Check sheet for the modelled part. Datum: model origin and axes. Units: mm. A direction names the side the tool comes from. Give positions to 0.01 mm unless a question says otherwise; leave off trailing zeros. Loops run counter-clockwise (first coordinate to the right, second up) from the corner with the lowest first, then second, coordinate; pieces in that order, holes last. Notation, with made-up numbers: (-7, 23.5) - (52, 23.5) arc R9 ccw to (52, 29.5) - close; hole circle Ø8 at (83, -22). An arc over 180 degrees is marked (long way). Answer in a Markdown table with one row per item. Add a question column.
(1) Draft check along Z on faces 1 (the face through (0, 0, -1.778)), 2 (the face through (1.433, 8.476, -2.711)), 3 (the face through (0.95, 0.3, 36.53)), 4 (the face through (-1.433, -8.476, -2.711)). Enter one of: released by +Z, released by -Z, zero draft, split by the parting line, or undercut.
(2) Go/stop test with flat-tipped pins: P1, Ø4, axis at y = -8.5, z = 24.5, coming from the +X side; P2, Ø1.7, axis at y = 9.11, z = -2.79, coming from the +X side; P3, Ø3, axis at x = -9, z = 13.5, coming from the -Y side; P4, Ø5, axis at y = 6.5, z = 34.5, coming from the +X side. Record where each tip stops, or that it passes through.
(3) Set-up check for faces 5 (the face through (1, 1, 32.715)), 6 (the face through (-1.27, -9, -1)), 7 (the face through (0, 0, 40.97)): record each of +Z, -Z, +X, -X, +Y, -Y from which the full face is reachable in a straight line by a thin tool's end or side.
(4) Sectioned sample at A-A on z = 14.5. Enter the section's corners in (x, y), then the cut area to 3 significant figures.
(5) Thickness scan on L1, parallel to Y at x = 0, z = 0.35; L2, parallel to Z at x = 3.75, y = 10; L3, parallel to X at y = -0.5, z = 6. Record the ranges inside material, lowest first.
from build123d import *

# Parameters (mm, degrees)
SKETCH1_R           = 12.192
BOSS_EXTRUDE1_DEPTH = 30.8102
SKETCH2_R           = 0.99695
BOSS_EXTRUDE3_DEPTH = 10.16
SKETCH6_R           = 3.2004
BOSS_EXTRUDE4_DEPTH = 1.905
FILLET2_R           = 0.508
FILLET3_R           = 1.27
SKETCH7_R           = 11.7094
CUT_EXTRUDE1_DEPTH  = 1.016
SKETCH10_R          = 3.2258
BOSS_EXTRUDE5_DEPTH = 2.794
FILLET4_R           = 0.889
SKETCH11_W          = 0.3302
SKETCH11_H          = 2.1082
BOSS_EXTRUDE6_DEPTH = 5.08
SKETCH12_R          = 0.635
CUT_EXTRUDE2_DEPTH  = 0.3302
CIRPATTERN1_COUNT   = 2


with BuildPart() as part:
    # Sketch1 → Boss-Extrude1 (new body)
    with BuildSketch(Plane.XY):
        Circle(SKETCH1_R)
    extrude(amount=BOSS_EXTRUDE1_DEPTH)

    # Sketch2 → Boss-Extrude3 (add)
    with BuildSketch(Plane.XY.offset(30.8102)):
        Circle(SKETCH2_R)
    extrude(amount=BOSS_EXTRUDE3_DEPTH)

    # Sketch6 → Boss-Extrude4 (add)
    with BuildSketch(Plane.XY.offset(30.8102)):
        Circle(SKETCH6_R)
    extrude(amount=BOSS_EXTRUDE4_DEPTH)

    # Fillet2
    fillet2_edges = [part.edges().sort_by_distance(p)[0] for p in [
        (-0.99695, 0, 40.9702),
    ]]
    fillet(fillet2_edges, radius=FILLET2_R)

    # Fillet3
    fillet3_edges = [part.edges().sort_by_distance(p)[0] for p in [
        (-12.192, 0, 30.8102),
    ]]
    fillet(fillet3_edges, radius=FILLET3_R)

    # Sketch7 → Cut-Extrude1 (cut)
    with BuildSketch(Plane(origin=(0, 0, 0), x_dir=(-1, 0, 0), z_dir=(0, 0, -1))):
        Circle(SKETCH7_R)
    extrude(amount=-CUT_EXTRUDE1_DEPTH, mode=Mode.SUBTRACT)

    # Sketch10 → Boss-Extrude5 (add)
    with BuildSketch(Plane(origin=(0, 0, 1.016), x_dir=(-1, 0, 0), z_dir=(0, 0, -1))):
        Circle(SKETCH10_R)
    extrude(amount=BOSS_EXTRUDE5_DEPTH)

    # Fillet4
    fillet4_edges = [part.edges().sort_by_distance(p)[0] for p in [
        (3.2258, 0, -1.778),
    ]]
    fillet(fillet4_edges, radius=FILLET4_R)

    # Sketch11 → Boss-Extrude6 (add)
    with BuildSketch(Plane(origin=(0, 0, 1.016), x_dir=(-1, 0, 0), z_dir=(0, 0, -1))):
        with Locations((1.4351, -9.1059)):
            Rectangle(SKETCH11_W, SKETCH11_H)
    boss_extrude6 = extrude(amount=BOSS_EXTRUDE6_DEPTH)

    # Sketch12 → Cut-Extrude2 (cut)
    with BuildSketch(Plane(origin=(-1.27, 0, 0), x_dir=(0, 0, -1), z_dir=(1, 0, 0))):
        with Locations((2.794, -9.1059)):
            Circle(SKETCH12_R)
        Polygon((3.302, -8.0518), (4.064, -8.8138), (4.064, -8.0518), align=None)
        Polygon((4.064, -9.398), (3.302, -10.16), (4.064, -10.16), align=None)
    cut_extrude2 = extrude(amount=-CUT_EXTRUDE2_DEPTH, mode=Mode.SUBTRACT)

    # CirPattern1: Boss-Extrude6, Cut-Extrude2 ×2 about axis
    cirpattern1_axis = Axis((0, 0, 0), (0, 0, 1))
    for i in range(1, CIRPATTERN1_COUNT):
        add(boss_extrude6.rotate(cirpattern1_axis, i * 360 / CIRPATTERN1_COUNT))
        add(cut_extrude2.rotate(cirpattern1_axis, i * 360 / CIRPATTERN1_COUNT), mode=Mode.SUBTRACT)


solid = part.part
Reply:
| question | item | result |
|---|---|---|
| 1 | face 1 | released by -Z |
| 1 | face 2 | undercut |
| 1 | face 3 | zero draft |
| 1 | face 4 | undercut |
| 2 | P1 | x = 10.31 |
| 2 | P2 | x = 1.6 |
| 2 | P3 | y = -9.61 |
| 2 | P4 | through |
| 3 | face 5 | +Z |
| 3 | face 6 | -Z |
| 3 | face 7 | +Z, +X, -X, +Y, -Y |
| 4 | outline | circle Ø24.38 at (0, 0) |
| 4 | area | 467 mm^2 |
| 5 | L1 | -12.19 to -11.71, -3.23 to 3.23, 11.71 to 12.19 |
| 5 | L2 | 1.02 to 30.81 |
| 5 | L3 | -12.18 to 12.18 |
